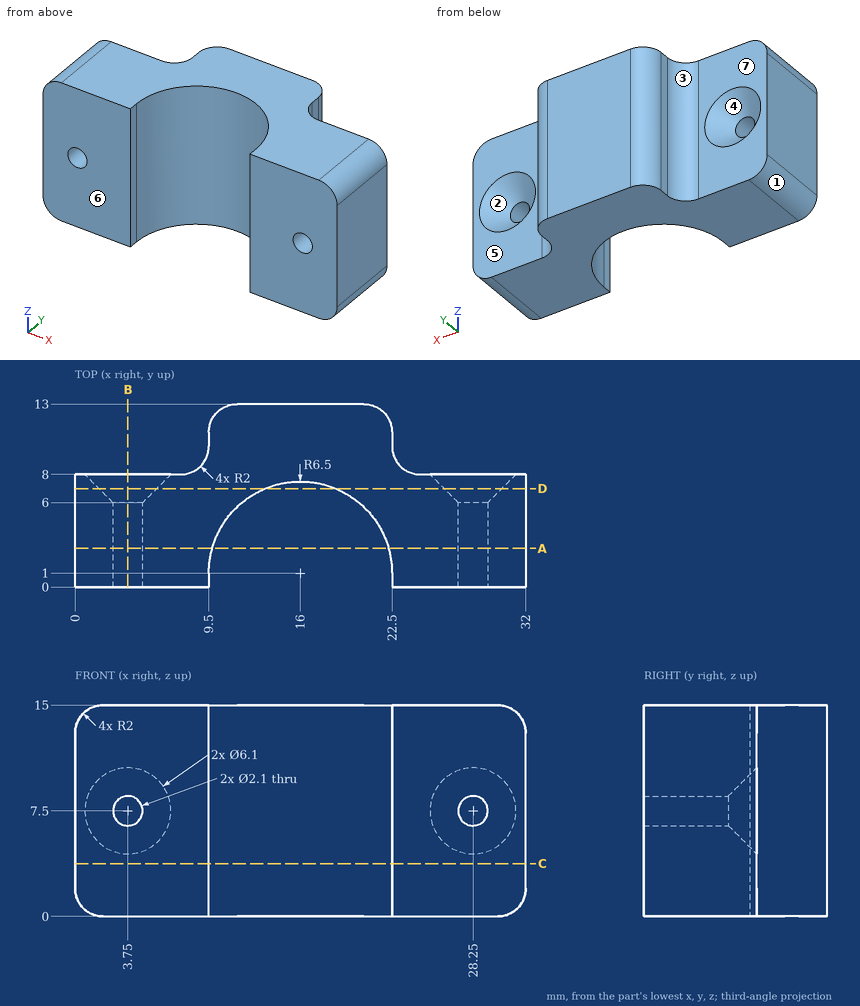
Geometry: see drawing. Coordinates: mm, zero at the bounding-box minimum. A direction names the side the tool comes from. Give positions to 0.01 mm unless a question says otherwise; leave off trailing zeros. Loops run counter-clockwise (first coordinate to the right, second up) from the corner with the lowest first, then second, coordinate; pieces in that order, holes last. Notation, with made-up numbers: (59.25, 76) -> (110.25, 76) arc R24 cw to (110.25, 101) -> close; hole circle Ø6 at (87, 24.5). An arc over 180 degrees is marked (long way). Answer as a JSON object with one key per item and string values. Group by question number.
Item 1: Cut plane A-A, the plane y = 2.75. Return the cut outline in (x, z).
Item 2: Cut plane B-B, the plane x = 3.75. Return the cut outline in (y, z).
Item 3: Cut plane D-D, the plane y = 7. Return the cut outline in (x, z), and give its area (3 significant figures).
Item 4: Line query: probe 1 along Z at (x, y) = (28.25, 4.35); probe 2 along X at (y, z) = (10.25, 13.75); probe 3 along Y at (x, z) = (25, 2.25). Output: solid intervals per line, ascending.
Item 5: Pull-direction query (Z, two-part tool) for the marked faces 1, 2, 3 and 4; classes: released by +Z, released by -Z, zero draft, split by the parting line, or undercut.
Item 6: Cut plane C-C, the plane z = 3.75. Return the cut outline in (x, y).
Item 7: Reachability of the marked faces 5, 6 and 7 from +Z, -Z, +X, -X, +Y, -Y: full face, straight path, thin tool, end or side. Return the list, or none.
Item 8: Pin query (flat end, axial travel): P1, Ø1, axis at x = 12.5, y = 6, coming from the +Z side; P2, Ø2, axis at x = 27.5, y = 10, coming from the -Z side; P3, Ø3, axis at x = 18, z = 7, coming from the -Y side; P4, Ø6, axis at x = 4.5, z = 9, coming from the +Y side. Return the tip coordinate at first contact, or that it passes through.
Checks:
{
 "1": {"outline": "(0, 2) arc R2 ccw to (2, 0) -> (9.74, 0) -> (9.74, 15) -> (2, 15) arc R2 ccw to (0, 13) -> close; (22.26, 0) -> (30, 0) arc R2 ccw to (32, 2) -> (32, 13) arc R2 ccw to (30, 15) -> (22.26, 15) -> close; hole circle Ø2.1 at (3.75, 7.5); hole circle Ø2.1 at (28.25, 7.5)"},
 "2": {"outline": "(0, 0) -> (8, 0) -> (8, 4.45) -> (6, 6.45) -> (0, 6.45) -> close; (0, 8.55) -> (6, 8.55) -> (8, 10.55) -> (8, 15) -> (0, 15) -> close"},
 "3": {"outline": "(0, 2) arc R2 ccw to (2, 0) -> (13.5, 0) -> (13.5, 15) -> (2, 15) arc R2 ccw to (0, 13) -> close; (18.5, 0) -> (30, 0) arc R2 ccw to (32, 2) -> (32, 13) arc R2 ccw to (30, 15) -> (18.5, 15) -> close; hole circle Ø4.1 at (3.75, 7.5); hole circle Ø4.1 at (28.25, 7.5)", "area": "375 mm²"},
 "4": {"probe 1": "z = 0 to 6.45, 8.55 to 15", "probe 2": "x = 9.5 to 22.5", "probe 3": "y = 0 to 8"},
 "5": {"face 1": "released by -Z", "face 2": "undercut", "face 3": "zero draft", "face 4": "undercut"},
 "6": {"outline": "(0, 0) -> (9.5, 0) -> (9.5, 1) arc R6.5 cw to (22.5, 1) -> (22.5, 0) -> (32, 0) -> (32, 8) -> (24.5, 8) arc R2 cw to (22.5, 10) -> (22.5, 11) arc R2 ccw to (20.5, 13) -> (11.5, 13) arc R2 ccw to (9.5, 11) -> (9.5, 10) arc R2 cw to (7.5, 8) -> (0, 8) -> close"},
 "7": {"face 5": "+Z, -Z, +X, +Y", "face 6": "+Z, -Z, +X, -X, -Y", "face 7": "+Z, -Z, -X, +Y"},
 "8": {"P1": "stops at z = 15", "P2": "passes through", "P3": "stops at y = 6.48", "P4": "stops at y = 8"}
}
